Here's how the part is built. I have some questions about the finished solid (model axes, mm). A direction names the side the tool comes from. Give positions to 0.01 mm unless a question says otherwise; leave off trailing zeros. Loops run counter-clockwise (first coordinate to the right, second up) from the corner with the lowest first, then second, coordinate; pieces in that order, holes last. Notation, with made-up numbers: (19, 63) - (78, 63) arc R4 ccw to (78, 67) - close; hole circle Ø6 at (-0.5, 28.5). An arc over 180 degrees is marked (long way). Use one line per item in the form item = value.
from build123d import *

# Parameters (mm, degrees)
SKETCH1_W           = 12.7
SKETCH1_H           = 3.4036
BOSS_EXTRUDE1_DEPTH = 6.35


with BuildPart() as part:
    # Sketch1 → Boss-Extrude1 (new body)
    with BuildSketch(Plane.XY):
        with BuildLine():
            Line((8603.455921527, 2991.548549024), (8603.455921527, 2951.939177286))
            Line((8603.455921527, 2951.939177286), (8610.440921527, 2951.939177286))
            ThreePointArc((8610.440921527, 2951.939177286), (8612.685985557, 2951.009241316), (8613.615921527, 2948.764177286))
            Line((8613.615921527, 2948.764177286), (8613.615921527, 2939.239177286))
            ThreePointArc((8613.615921527, 2939.239177286), (8612.685985557, 2936.994113255), (8610.440921527, 2936.064177286))
            Line((8610.440921527, 2936.064177286), (8603.455921527, 2936.064177286))
            Line((8603.455921527, 2936.064177286), (8603.455921527, 2909.495777286))
            ThreePointArc((8603.455921527, 2909.495777286), (8604.928940103, 2905.939595862), (8608.485121527, 2904.466577286))
            Line((8608.485121527, 2904.466577286), (8608.485121527, 2907.870177286))
            Line((8608.485121527, 2907.870177286), (8621.185121527, 2907.870177286))
            Line((8621.185121527, 2907.870177286), (8621.185121527, 2904.466577286))
            Line((8621.185121527, 2904.466577286), (8666.752721527, 2904.466577286))
            Line((8666.752721527, 2904.466577286), (8666.752721527, 2907.870177286))
            Line((8666.752721527, 2907.870177286), (8679.452721527, 2907.870177286))
            Line((8679.452721527, 2907.870177286), (8679.452721527, 2904.466577286))
            ThreePointArc((8679.452721527, 2904.466577286), (8683.008902951, 2905.939595862), (8684.481921527, 2909.495777286))
            Line((8684.481921527, 2909.495777286), (8684.481921527, 2936.064177286))
            Line((8684.481921527, 2936.064177286), (8677.496921527, 2936.064177286))
            ThreePointArc((8677.496921527, 2936.064177286), (8675.251857497, 2936.994113255), (8674.321921527, 2939.239177286))
            Line((8674.321921527, 2939.239177286), (8674.321921527, 2948.764177286))
            ThreePointArc((8674.321921527, 2948.764177286), (8675.251857497, 2951.009241316), (8677.496921527, 2951.939177286))
            Line((8677.496921527, 2951.939177286), (8684.481921527, 2951.939177286))
            Line((8684.481921527, 2951.939177286), (8684.481921527, 2991.548549024))
            ThreePointArc((8684.481921527, 2991.548549024), (8683.008902951, 2995.104730448), (8679.452721527, 2996.577749024))
            Line((8679.452721527, 2996.577749024), (8679.452721527, 2993.174149024))
            Line((8679.452721527, 2993.174149024), (8666.752721527, 2993.174149024))
            Line((8666.752721527, 2993.174149024), (8666.752721527, 2996.577749024))
            Line((8666.752721527, 2996.577749024), (8621.185121527, 2996.577749024))
            Line((8621.185121527, 2996.577749024), (8621.185121527, 2993.174149024))
            Line((8621.185121527, 2993.174149024), (8608.485121527, 2993.174149024))
            Line((8608.485121527, 2993.174149024), (8608.485121527, 2996.577749024))
            ThreePointArc((8608.485121527, 2996.577749024), (8604.928940103, 2995.104730448), (8603.455921527, 2991.548549024))
        make_face()
        with Locations((8623.013921527, 2917.928577286)):
            Rectangle(SKETCH1_W, SKETCH1_H, mode=Mode.SUBTRACT)
        with Locations((8664.923921527, 2917.928577286)):
            Rectangle(SKETCH1_W, SKETCH1_H, mode=Mode.SUBTRACT)
        with Locations((8664.923921527, 2979.193377286)):
            Rectangle(SKETCH1_W, SKETCH1_H, mode=Mode.SUBTRACT)
        with Locations((8623.013921527, 2979.193377286)):
            Rectangle(SKETCH1_W, SKETCH1_H, mode=Mode.SUBTRACT)
    extrude(amount=BOSS_EXTRUDE1_DEPTH)


solid = part.part
(1) For faces 4 (the flat face through (8679.453, 2995, 3)), 5 (the flat face through (8607, 2936.064, 3)), 6 (the flat face through (8623, 2916.227, 3)), which set-ups out of +Z, -Z, +X, -X, +Y, -Y let a thin tool reach every point of the face, with its end or its side?
Geometry says:
face_4 = +Z, -Z, +Y
face_5 = +Z, -Z, -X
face_6 = +Z, -Z
(2) If we section it at A-A (y = 2979.5): List the corners of the cut face in (x, z) for me.
Geometry says:
outline = (8603.46, 0) - (8616.66, 0) - (8616.66, 6.35) - (8603.46, 6.35) - close; (8629.36, 0) - (8658.57, 0) - (8658.57, 6.35) - (8629.36, 6.35) - close; (8671.27, 0) - (8684.48, 0) - (8684.48, 6.35) - (8671.27, 6.35) - close
(3) Thinking about a two-plate mould opening in X: for faces 1 (the flat face through (8684.482, 2971, 3)), 2 (the cylindrical face through (8612.661, 2951.034, 3.131)), 3 (the flat face through (8615, 2907.87, 3)), which applies, pulls with the +X half, pulls with the -X half, needs draft (parallel to the pull), parting line crosses it, or undercut?
Geometry says:
face_1 = pulls with the +X half
face_2 = pulls with the -X half
face_3 = undercut
(4) If we section it at C-C (z = 1): Give the number of separate pieces and of enclosed holes in the cut face, plus the area to 3 significant figures.
Geometry says:
separate_pieces = 1
enclosed_holes = 4
area = 6,780 mm²
(5) If we section it at B-B (x = 8619): List the corners of the cut face in (y, z) for me.
Geometry says:
outline = (2907.87, 0) - (2916.23, 0) - (2916.23, 6.35) - (2907.87, 6.35) - close; (2919.63, 0) - (2977.49, 0) - (2977.49, 6.35) - (2919.63, 6.35) - close; (2980.9, 0) - (2993.17, 0) - (2993.17, 6.35) - (2980.9, 6.35) - close
(6) If I drill on probe 1 along Y at (x, z) = (8617.5, 4.5); probe 2 along Y at (x, z) = (8629, 5); probe 3 along Y at (x, z) = (8609, 0.5), over which ranges is the centre line in solid material (lowest first)?
Geometry says:
probe_1 = 2907.87 to 2916.23, 2919.63 to 2977.49, 2980.9 to 2993.17
probe_2 = 2904.47 to 2916.23, 2919.63 to 2977.49, 2980.9 to 2996.58
probe_3 = 2907.87 to 2936.06, 2951.94 to 2993.17
(7) For P1, Ø3.5, axis at y = 2905.5, z = 1.5, coming from the +X side; P2, Ø1.5, axis at x = 8674.5, z = 5, coming from the -Y side; P3, Ø3.5, axis at y = 2905.5, z = 4, coming from the -X side, each with a flat end and sliding along its axis, tell me the tip position at first contact or that it passes through.
Geometry says:
P1 = 8683.95
P2 = 2907.87
P3 = 8603.99
